```python
from build123d import *

# Parameters (mm, degrees)
SKETCH1_W           = 40
SKETCH1_H           = 61
SKETCH1_W_2         = 34
SKETCH1_H_2         = 55
BOSS_EXTRUDE1_DEPTH = 72.2
FILLET1_R           = 8
FILLET2_R           = 8
SKETCH2_R           = 1.45
BOSS_EXTRUDE2_DEPTH = 4
SKETCH3_W           = 24
SKETCH3_H           = 44.7
CUT_EXTRUDE1_DEPTH  = 4
BOSS_EXTRUDE3_DEPTH = 30
FILLET3_R           = 15
FILLET4_R           = 15
SKETCH6_R           = 2
CUT_EXTRUDE2_DEPTH  = 5
SKETCH8_R           = 1.505
CUT_EXTRUDE3_DEPTH  = 5
FILLET5_R           = 2
BOSS_EXTRUDE5_DEPTH = 3
FILLET7_R           = 5
SKETCH12_R          = 1.525
CUT_EXTRUDE4_DEPTH  = 3
CUT_EXTRUDE5_START  = -3
SKETCH13_R          = 1.525
CUT_EXTRUDE5_DEPTH  = 3
BOSS_EXTRUDE6_DEPTH = 4


with BuildPart() as part:
    # Sketch1 → Boss-Extrude1 (new body)
    with BuildSketch(Plane(origin=(0, 0, 0), x_dir=(1, 0, 0), z_dir=(0, 1, 0))):
        with Locations((20, 30.5)):
            Rectangle(SKETCH1_W, SKETCH1_H)
        with Locations((20, 30.5)):
            Rectangle(SKETCH1_W_2, SKETCH1_H_2, mode=Mode.SUBTRACT)
    extrude(amount=BOSS_EXTRUDE1_DEPTH)

    # Fillet1
    fillet1_edges = [part.edges().sort_by_distance(p)[0] for p in [
        (37, 36.1, -3),
        (37, 36.1, -58),
        (3, 36.1, -58),
        (3, 36.1, -3),
    ]]
    fillet(fillet1_edges, radius=FILLET1_R)

    # Fillet2
    fillet2_edges = [part.edges().sort_by_distance(p)[0] for p in [
        (0, 36.1, -61),
        (40, 36.1, -61),
        (40, 36.1, 0),
        (0, 36.1, 0),
    ]]
    fillet(fillet2_edges, radius=FILLET2_R)

    # Sketch2 → Boss-Extrude2 (add)
    # profile 1 of 2: a face of its own
    with BuildSketch(Plane(origin=(0, 27.5, 0), x_dir=(-1, 0, 0), z_dir=(0, -1, 0))):
        with BuildLine():
            ThreePointArc((-3.127033596, 51.42), (-5.869697865, 56.138403701), (-11, 58))
            Line((-11, 58), (-29, 58))
            ThreePointArc((-29, 58), (-34.130302135, 56.138403701), (-36.872966404, 51.42))
            Line((-36.872966404, 51.42), (-22.135286633, 51.42))
            Line((-22.135286633, 51.42), (-22.135286633, 57.223660853))
            Line((-22.135286633, 57.223660853), (-17.994848526, 57.223660853))
            Line((-17.994848526, 57.223660853), (-17.994848526, 51.42))
            Line((-17.994848526, 51.42), (-3.127033596, 51.42))
        make_face()
        with Locations(Location((-24.9, 54.8, 0), (0, 0, 90))):
            Circle(SKETCH2_R, mode=Mode.SUBTRACT)
        with Locations(Location((-15.1, 54.8, 0), (0, 0, 90))):
            Circle(SKETCH2_R, mode=Mode.SUBTRACT)
    # profile 2 of 2: a face of its own
    with BuildSketch(Plane(origin=(0, 27.5, 0), x_dir=(-1, 0, 0), z_dir=(0, -1, 0))):
        with BuildLine():
            ThreePointArc((-29, 3), (-34.130302135, 4.861596299), (-36.872966404, 9.58))
            Line((-36.872966404, 9.58), (-3.127033596, 9.58))
            ThreePointArc((-3.127033596, 9.58), (-5.869697865, 4.861596299), (-11, 3))
            Line((-11, 3), (-29, 3))
        make_face()
        with Locations(Location((-24.9, 6.2, 0), (0, 0, 90))):
            Circle(SKETCH2_R, mode=Mode.SUBTRACT)
        with Locations(Location((-15.1, 6.2, 0), (0, 0, 90))):
            Circle(SKETCH2_R, mode=Mode.SUBTRACT)
    extrude(amount=BOSS_EXTRUDE2_DEPTH)

    # Sketch3 → Cut-Extrude1 (cut)
    with BuildSketch(Plane.XY):
        with Locations((20, 49.85)):
            Rectangle(SKETCH3_W, SKETCH3_H)
    extrude(amount=-CUT_EXTRUDE1_DEPTH, mode=Mode.SUBTRACT)

    # Sketch5 → Boss-Extrude3 (add)
    with BuildSketch(Plane(origin=(0, 0, -55.65), x_dir=(-1, 0, 0), z_dir=(0, 0, -1))):
        Polygon((-40, 22.623135631), (-63, 8.644648184), (-63, -46.266055448), (-58, -46.266055448), (-58, 0), (-40, 0), align=None)
        Polygon((0, 22.623135631), (0, 0), (18, 0), (18, -46.266055448), (23, -46.266055448), (23, 8.644648184), align=None)
    extrude(amount=-BOSS_EXTRUDE3_DEPTH)

    # Fillet3
    fillet3_edges = [part.edges().sort_by_distance(p)[0] for p in [
        (60.5, -46.266055448, -55.65),
        (60.5, -46.266055448, -25.65),
    ]]
    fillet(fillet3_edges, radius=FILLET3_R - 0.0001)  # a hair under: the kernel refuses the full size

    # Fillet4
    fillet4_edges = [part.edges().sort_by_distance(p)[0] for p in [
        (-20.5, -46.266055448, -25.65),
        (-20.5, -46.266055448, -55.65),
    ]]
    fillet(fillet4_edges, radius=FILLET4_R - 0.0001)  # a hair under: the kernel refuses the full size

    # Sketch6 → Cut-Extrude2 (cut)
    with BuildSketch(Plane(origin=(63, 0, 0), x_dir=(0, 0, -1), z_dir=(1, 0, 0))):
        with Locations((40.65, -31.266055448)):
            Circle(SKETCH6_R)
    extrude(amount=-CUT_EXTRUDE2_DEPTH, mode=Mode.SUBTRACT)

    # Sketch8 → Cut-Extrude3 (cut)
    with BuildSketch(Plane(origin=(63, 0, -67), x_dir=(0, 0, 1), z_dir=(-1, 0, 0))):
        with Locations((31.299747468, -26.316307979)):
            Circle(SKETCH8_R)
        with Locations((21.400252532, -26.316307979)):
            Circle(SKETCH8_R)
        with Locations((21.400252532, -36.215802916)):
            Circle(SKETCH8_R)
        with Locations((31.299747468, -36.215802916)):
            Circle(SKETCH8_R)
    extrude(amount=CUT_EXTRUDE3_DEPTH, mode=Mode.SUBTRACT)

    # Fillet5
    fillet5_edges = [part.edges().sort_by_distance(p)[0] for p in [
        (63, -11.310753632, -25.65),
        (51.5, 15.633891908, -25.65),
        (51.5, 15.633891908, -55.65),
        (63, -11.310753632, -55.65),
        (-11.5, 15.633891908, -25.65),
        (-11.5, 15.633891908, -55.65),
        (63, -41.872686455, -30.043368993),
        (63, -41.872686455, -51.256631007),
        (-23, -11.310753632, -55.65),
        (-23, -11.310753632, -25.65),
        (-23, -41.872686455, -51.256631007),
        (-23, -41.872686455, -30.043368993),
    ]]
    fillet(fillet5_edges, radius=FILLET5_R)

    # Sketch11 → Boss-Extrude5 (add)
    with BuildSketch(Plane(origin=(0, 69.2, 0), x_dir=(1, 0, 0), z_dir=(0, 1, 0))):
        with BuildLine():
            ThreePointArc((10, 57.937253933), (5, 55.291502622), (3, 50))
            Line((3, 50), (10, 50))
            Line((10, 50), (10, 57.937253933))
        make_face()
        with BuildLine():
            Line((30, 50), (37, 50))
            ThreePointArc((37, 50), (35, 55.291502622), (30, 57.937253933))
            Line((30, 57.937253933), (30, 50))
        make_face()
    extrude(amount=-BOSS_EXTRUDE5_DEPTH)

    # Fillet7
    fillet7_edges = [part.edges().sort_by_distance(p)[0] for p in [
        (5, 66.2, -55.291502622),
        (35, 66.2, -55.291502622),
    ]]
    fillet(fillet7_edges, radius=FILLET7_R)

    # Sketch12 → Cut-Extrude4 (cut)
    with BuildSketch(Plane(origin=(3, 0, 0), x_dir=(0, 0, -1), z_dir=(1, 0, 0))):
        with Locations((44.95, 67.2)):
            Circle(SKETCH12_R)
    extrude(amount=-CUT_EXTRUDE4_DEPTH, mode=Mode.SUBTRACT)

    # Sketch13 → Cut-Extrude5 (cut)
    with BuildSketch(Plane.ZY.offset(-37).offset(CUT_EXTRUDE5_START)):
        with Locations(Location((-44.95, 67.2, 0), (0, 0, 180))):
            Circle(SKETCH13_R)
    extrude(amount=CUT_EXTRUDE5_DEPTH, mode=Mode.SUBTRACT)

    # Sketch14 → Boss-Extrude6 (add)
    with BuildSketch(Plane.XZ.offset(-23.5)):
        Polygon((3, -17.922275148), (10, -9.58), (3, -9.58), align=None)
        Polygon((37, -17.922275148), (30, -9.58), (37, -9.58), align=None)
    extrude(amount=-BOSS_EXTRUDE6_DEPTH)


solid = part.part
```
Verification items for the finished model (mm, model axes). A direction names the side the tool comes from. Coordinates: 2 decimals unless noted, no trailing zeros. Write each loop counter-clockwise with the first axis right and the second up, starting at its lowest first coordinate (ties: lowest second). Pieces come first, ordered by that corner, then holes. Notation, with made-up numbers: M -37.5,38.5 L 5.5,38.5 A27 cw 5.5,70.5 Z; hole C 7,-24 d7. An arc over 180 degrees is marked long. Answer as a JSON object with one key per item and string values. Group by question number.
(1) Tool access check on faces 3 (the face through (37.4, 0, -37.7)), 4 (the face through (20, 12, -3)), 5 (the face through (60.54, -25.3, -36.81)). Record the directions out of +Z, -Z, +X, -X, +Y, -Y that give a thin tool (end or side, any length) a straight path to the whole face; none if there is none.
(2) Cross-section at B-B, the plane x = 24.9. Record the cut outline in (y, z), and give its area (3 significant figures).
(3) Cross-section at D-D, the plane z = -6.2. Record the cut outline in (x, y).
(4) Cross-section at C-C, the plane y = 34. Record the cut outline in (x, z).
(5) Cross-section at A-A, the plane z = -22. Record the cut outline in (x, y).
(6) Material ranges on line 1 (X direction, y = -3, z = -29); line 2 (X direction, y = 62, z = -21.5); line 3 (X direction, y = 26.5, z = -6.2), recorded low to high.
(7) Release check for a two-part mould opening along X. For faces 1 (the face through (51, 1, -25.65)), 2 (the face through (5.406, 11.914, -5.281)) record: +X half, -X half, draft (parallel to the pull), parting line (faces both ways), or undercut.
(8) Gauge pin test, flat ends, axial feed: pin 1 (6 mm diameter, centred on x = 46, z = -26.5, fed in from -Y); pin 2 (1.5 mm diameter, centred on y = 38.5, z = -23.5, fed in from -X); pin 3 (1.5 mm diameter, centred on y = 16.5, z = -38, fed in from +X). Record the tip position at first contact, or that the pin passes through.
Reply:
{
 "1": {"face 3": "+Z, -Z, -Y", "face 4": "-Y", "face 5": "+X"},
 "2": {"outline": "M 0,-61 L 72.2,-61 L 72.2,-58 L 27.5,-58 L 27.5,-56.25 L 23.5,-56.25 L 23.5,-58 L 0,-58 Z; M 0,-3 L 23.5,-3 L 23.5,-4.75 L 27.5,-4.75 L 27.5,0 L 0,0 Z; M 23.5,-53.35 L 27.5,-53.35 L 27.5,-51.42 L 23.5,-51.42 Z; M 23.5,-9.58 L 27.5,-9.58 L 27.5,-7.65 L 23.5,-7.65 Z", "area": "329 mm²"},
 "3": {"outline": "M 0.21,0 L 4.6,0 L 4.6,23.5 L 13.65,23.5 L 13.65,27.5 L 4.6,27.5 L 4.6,72.2 L 0.21,72.2 Z; M 16.55,23.5 L 23.45,23.5 L 23.45,27.5 L 16.55,27.5 Z; M 26.35,23.5 L 35.4,23.5 L 35.4,0 L 39.79,0 L 39.79,72.2 L 35.4,72.2 L 35.4,27.5 L 26.35,27.5 Z"},
 "4": {"outline": "M 0,-53 A8 ccw 8,-61 L 32,-61 A8 ccw 40,-53 L 40,-8 A8 ccw 32,0 L 32,-3.58 A8 cw 37,-11 L 37,-50 A8 cw 29,-58 L 11,-58 A8 cw 3,-50 L 3,-11 A8 cw 8,-3.58 L 8,0 A8 ccw 0,-8 Z"},
 "5": {"outline": "M 0,0 L 3,0 L 3,72.2 L 0,72.2 Z; M 37,0 L 40,0 L 40,72.2 L 37,72.2 Z"},
 "6": {"line 1": "-23 to -18, 58 to 63", "line 2": "0 to 3, 37 to 40", "line 3": "0.21 to 13.65, 16.55 to 23.45, 26.35 to 39.79"},
 "7": {"face 1": "draft", "face 2": "undercut"},
 "8": {"pin 1": "y = 0", "pin 2": "x = 0", "pin 3": "x = 51.31"}
}
